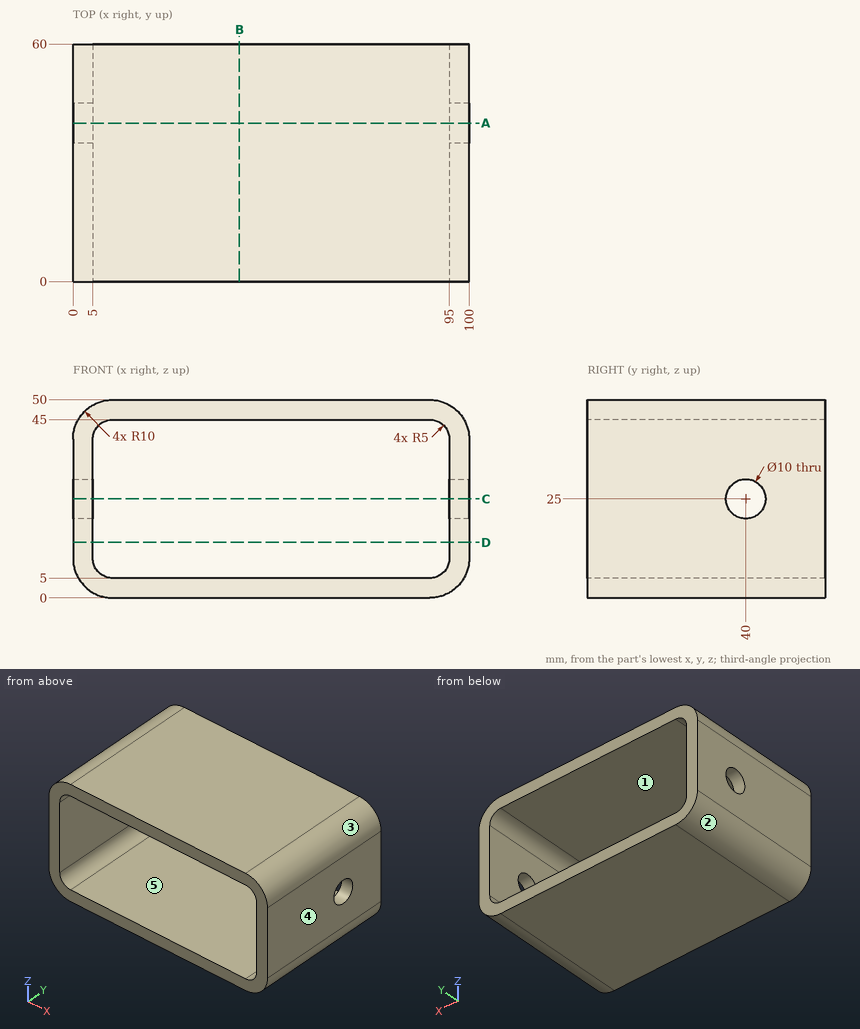
Geometry check sheet. Reference: drawing and pictorial views, mm from the part's lowest x, y, z. A direction names the side the tool comes from. Give positions to 0.01 mm unless a question says otherwise; leave off trailing zeros. Order: outer loops, then holes, each group sorted by start corner. A loop starts at its lowest first (then second) coordinate and runs counter-clockwise, first axis right, second up. Notation, with made-up numbers: M 27,20.25 L 43,20.25 A22 ccw 43,50.25 Z; hole C -6,-0.5 d4. An arc over 180 degrees is marked long. Return JSON: item names as keys, results as strings. Group by question number.
1) Go/stop test with flat-tipped pins: pin 1 Ø6 at (y, z) = (40, 25) entering from -X; pin 2 Ø13 at (y, z) = (40, 25) entering from -X. Record where each tip stops, or that it passes through.
2) Section check B-B on x = 42. Record the cut outline in (y, z).
3) Section check A-A on y = 40. Record the cut outline in (x, z).
4) Section check C-C on z = 25. Record the cut outline in (x, y).
5) Scan lines: line 1 (X direction, y = 57.5, z = 11); line 2 (Z direction, x = 90.5, y = 23.5); line 3 (Y direction, x = 97, z = 25). Record each from-to range of solid material in increasing order.
6) Section check D-D on z = 14. Record the cut outline in (x, y), and give its area (3 significant figures).
7) Access from +Z, -Z, +X, -X, +Y, -Y to the whole of each face (thin tool, end or side, straight path). Record for the marked faces 4 and 5.
8) Mould release check, pull along X, two halves, no side actions. Record for the marked faces 1, 2 and 3: pulls with the +X half, pulls with the -X half, needs draft (parallel to the pull), parting line crosses it, or undercut.
Answer block:
{
 "1": {"pin 1": "passes through", "pin 2": "stops at x = 0"},
 "2": {"outline": "M 0,0 L 60,0 L 60,5 L 0,5 Z; M 0,45 L 60,45 L 60,50 L 0,50 Z"},
 "3": {"outline": "M 0,10 A10 ccw 10,0 L 90,0 A10 ccw 100,10 L 100,20 L 95,20 L 95,10 A5 cw 90,5 L 10,5 A5 cw 5,10 L 5,20 L 0,20 Z; M 0,30 L 5,30 L 5,40 A5 cw 10,45 L 90,45 A5 cw 95,40 L 95,30 L 100,30 L 100,40 A10 ccw 90,50 L 10,50 A10 ccw 0,40 Z"},
 "4": {"outline": "M 0,0 L 5,0 L 5,35 L 0,35 Z; M 0,45 L 5,45 L 5,60 L 0,60 Z; M 95,0 L 100,0 L 100,35 L 95,35 Z; M 95,45 L 100,45 L 100,60 L 95,60 Z"},
 "5": {"line 1": "x = 0 to 5, 95 to 100", "line 2": "z = 0.01 to 5.03, 44.97 to 49.99", "line 3": "y = 0 to 35, 45 to 60"},
 "6": {"outline": "M 0,0 L 5,0 L 5,60 L 0,60 Z; M 95,0 L 100,0 L 100,60 L 95,60 Z", "area": "600 mm^2"},
 "7": {"face 4": "+Z, -Z, +X, +Y, -Y", "face 5": "+Y, -Y"},
 "8": {"face 1": "undercut", "face 2": "pulls with the -X half", "face 3": "pulls with the +X half"}
}
